Here's how the part is built. I have some questions about the finished solid (model axes, mm). Face numbers are marked on the shaded views. A direction names the side the tool comes from. Give positions to 0.01 mm unless a question says otherwise; leave off trailing zeros. Loops run counter-clockwise (first coordinate to the right, second up) from the corner with the lowest first, then second, coordinate; pieces in that order, holes last. Notation, with made-up numbers: (8, -35) - (39, -35) arc R33 ccw to (39, 4) - close; hole circle Ø9 at (17, -21.75). An arc over 180 degrees is marked (long way). Use one line per item in the form item = value.
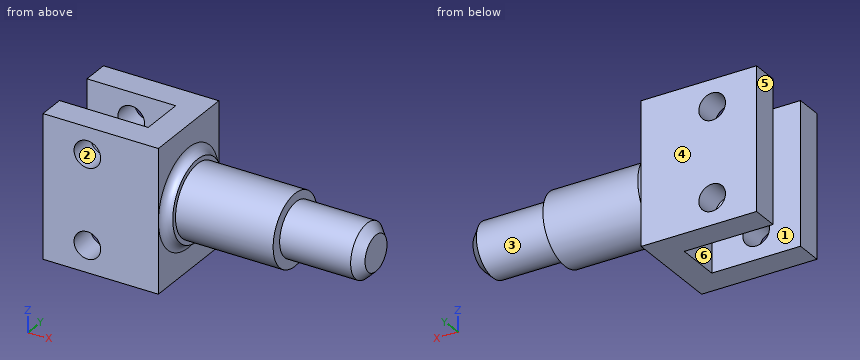
from build123d import *

# Parameters (mm, degrees)
EXTRUDE_1_DEPTH     = 16
SKETCH_2_R          = 1.5
CUT_EXTRUDE_1_DEPTH = 16
SKETCH_3_R          = 4.5
EXTRUDE_2_DEPTH     = 1
FILLET_1_R          = 1
SKETCH_4_R          = 4
EXTRUDE_3_DEPTH     = 11
SKETCH_5_R          = 3
EXTRUDE_4_DEPTH     = 9
CHAMFER_1_SIZE      = 1


with BuildPart() as part:
    # 草图1 → 凸台-拉伸1 (new body)
    with BuildSketch(Plane.XY):
        Polygon((0, 0), (13, 0), (13, 11), (0, 11), (0, 8), (10, 8), (10, 3), (0, 3), align=None)
    extrude(amount=EXTRUDE_1_DEPTH)

    # 草图2 → 切除-拉伸1 (cut)
    with BuildSketch(Plane(origin=(0, 11, 0), x_dir=(1, 0, 0), z_dir=(0, 1, 0))):
        with Locations(Location((5, -3, 0), (0, 0, 270))):
            Circle(SKETCH_2_R)
        with Locations(Location((5, -13, 0), (0, 0, 270))):
            Circle(SKETCH_2_R)
    extrude(amount=-CUT_EXTRUDE_1_DEPTH, mode=Mode.SUBTRACT)

    # 草图3 → 凸台-拉伸2 (add)
    with BuildSketch(Plane(origin=(13, 0, 0), x_dir=(0, 0, -1), z_dir=(1, 0, 0))):
        with Locations((-8, 5.5)):
            Circle(SKETCH_3_R)
    extrude(amount=EXTRUDE_2_DEPTH)

    # 圆角1
    fillet_1_edges = [part.edges().sort_by_distance(p)[0] for p in [
        (13, 5.5, 12.5),
    ]]
    fillet(fillet_1_edges, radius=FILLET_1_R - 0.0001)  # a hair under: the kernel refuses the full size

    # 草图4 → 凸台-拉伸3 (add)
    with BuildSketch(Plane(origin=(14, 0, 0), x_dir=(0, 0, -1), z_dir=(1, 0, 0))):
        with Locations((-8, 5.5)):
            Circle(SKETCH_4_R)
    extrude(amount=EXTRUDE_3_DEPTH)

    # 草图5 → 凸台-拉伸4 (add)
    with BuildSketch(Plane(origin=(25, 0, 0), x_dir=(0, 0, -1), z_dir=(1, 0, 0))):
        with Locations((-8, 5.683281664)):
            Circle(SKETCH_5_R)
    extrude(amount=EXTRUDE_4_DEPTH)

    # 倒角1
    chamfer_1_edges = [part.edges().sort_by_distance(p)[0] for p in [
        (34, 5.683281664, 11),
    ]]
    chamfer(chamfer_1_edges, length=CHAMFER_1_SIZE)


solid = part.part
(1) If we section it at B-B (z = 1): List the corners of the cut face in (x, y) for me.
Geometry says:
outline = (0, 0) - (13, 0) - (13, 11) - (0, 11) - (0, 8) - (10, 8) - (10, 3) - (0, 3) - close
(2) For the marked faces 1, 2 and 3, which set-ups out of +Z, -Z, +X, -X, +Y, -Y let a thin tool reach every point of the face, with its end or its side?
Geometry says:
face_1 = +Z, -Z, -X
face_2 = +Y, -Y
face_3 = +X
(3) If we section it at A-A (x = 5): List the corners of the cut face in (y, z) for me.
Geometry says:
outline = (0, 0) - (3, 0) - (3, 1.5) - (0, 1.5) - close; (0, 4.5) - (3, 4.5) - (3, 11.5) - (0, 11.5) - close; (0, 14.5) - (3, 14.5) - (3, 16) - (0, 16) - close; (8, 0) - (11, 0) - (11, 1.5) - (8, 1.5) - close; (8, 4.5) - (11, 4.5) - (11, 11.5) - (8, 11.5) - close; (8, 14.5) - (11, 14.5) - (11, 16) - (8, 16) - close
(4) Thinking about a two-plate mould opening in Y: for the marked faces 4, 5 and 6, which applies, pulls with the +Y half, pulls with the -Y half, needs draft (parallel to the pull), parting line crosses it, or undercut?
Geometry says:
face_4 = pulls with the +Y half
face_5 = needs draft
face_6 = undercut
(5) If we section it at C-C (z = 13): Give the number of separate pieces and of enclosed holes in the cut face, plus the area to 3 significant figures.
Geometry says:
separate_pieces = 3
enclosed_holes = 0
area = 75.3 mm²
(6) If I drill on probe 1 along X at (y, z) = (9.25, 13); probe 2 along Y at (x, z) = (2, 11.5); probe 3 along X at (y, z) = (9.5, 4.25), over which ranges is the centre line in solid material (lowest first)?
Geometry says:
probe_1 = 0 to 3.5, 6.5 to 13
probe_2 = 0 to 3, 8 to 11
probe_3 = 0 to 4.17, 5.83 to 13
(7) For P1, Ø1, axis at x = 26.5, y = 2.5, coming from the +Z side, with a flat end and sliding along its axis, tell me the tip position at first contact or that it passes through.
Geometry says:
P1 = 9.34
